Model file for the job. Use its own axes, mm. Give positions to 0.01 mm unless a question says otherwise; leave off trailing zeros. Loops run counter-clockwise (first coordinate to the right, second up) from the corner with the lowest first, then second, coordinate; pieces in that order, holes last. Notation, with made-up numbers: (4.5, 9) - (29.5, 9) arc R23 ccw to (29.5, 19) - close; hole circle Ø1 at (-0.5, -12.5). An arc over 180 degrees is marked (long way). Use a Markdown table: item, result.
from build123d import *

# Parameters (mm, degrees)
SKETCH_1_W      = 6
SKETCH_1_H      = 6
EXTRUDE_1_DEPTH = 20
HOLE_WIZARD_1_D = 2.5
HOLE_WIZARD_2_D = 2.5
CHAMFER_1_SIZE  = 0.3


with BuildPart() as part:
    # 草图1 → 凸台-拉伸1 (new, symmetric)
    with BuildSketch(Plane.XY):
        Rectangle(SKETCH_1_W, SKETCH_1_H)
    extrude(amount=EXTRUDE_1_DEPTH, both=True)

    # Hole Wizard 1 (through all)
    with Locations(Plane.ZY.offset(3)):
        with Locations((-15, 0), (5, 0)):
            Hole(HOLE_WIZARD_1_D / 2)

    # Hole Wizard 2 (through all)
    with Locations(Plane(origin=(0, 3, 0), x_dir=(1, 0, 0), z_dir=(0, 1, 0))):
        with Locations((0, 5), (0, -15)):
            Hole(HOLE_WIZARD_2_D / 2)

    # 倒角1
    chamfer_1_edges = [part.edges().sort_by_distance(p)[0] for p in [
        (-3, 0, 20),
        (0, -3, 20),
        (3, 0, 20),
        (0, -3, -20),
        (-3, 0, -20),
        (0, 3, -20),
        (3, 0, -20),
        (3, -3, 0),
        (-3, -3, 0),
        (-3, 3, 0),
        (3, 3, 0),
        (0, 3, 20),
    ]]
    chamfer(chamfer_1_edges, length=CHAMFER_1_SIZE)


solid = part.part
(1) Pin check, flat tip, straight feed: P1, Ø1, axis at y = 0, z = 5.5, coming from the +X side. Stop position of the tip, or through.
Computed:
| item | result |
|---|---|
| P1 | through |
(2) Drill centre lines: probe 1 along Z at (x, y) = (0, 1.85); probe 2 along X at (y, z) = (0.25, -5); probe 3 along Z at (x, y) = (1.5, 1). Where is each one in solid material? Low to high. Write a range as [from, to].
Computed:
| item | result |
|---|---|
| probe 1 | [-20, -6.25], [-3.75, 13.75], [16.25, 20] |
| probe 2 | [-3, -1.25], [1.25, 3] |
| probe 3 | [-20, -15.75], [-14.25, 4.25], [5.75, 20] |
(3) Slice it at B-B, the plane y = 0. Write the cut outline in (x, z).
Computed:
| item | result |
|---|---|
| outline | (-3, -19.7) - (-2.7, -20) - (2.7, -20) - (3, -19.7) - (3, -16.25) - (-3, -16.25) - close; (-3, -13.75) - (3, -13.75) - (3, 3.75) - (-3, 3.75) - close; (-3, 6.25) - (3, 6.25) - (3, 19.7) - (2.7, 20) - (-2.7, 20) - (-3, 19.7) - close; hole circle Ø2.5 at (0, -5); hole circle Ø2.5 at (0, 15) |
(4) Slice it at D-D, the plane y = -2. Write the cut outline in (x, z), plus the area to 3 significant figures.
Computed:
| item | result |
|---|---|
| outline | (-3, -19.7) - (-2.7, -20) - (2.7, -20) - (3, -19.7) - (3, 19.7) - (2.7, 20) - (-2.7, 20) - (-3, 19.7) - close; hole circle Ø2.5 at (0, -5); hole circle Ø2.5 at (0, 15) |
| area | 230 mm² |
(5) Mould opens along Z. For faces 1 (the cylindrical face through (0.16, -0.04, 13.76)), 2 (the cylindrical face through (0.04, 0.05, 6.25)), 3 (the flat face through (0, 3, 0)), 4 (the flat face through (0, 0, 20)) say: pulls with the +Z half, pulls with the -Z half, needs draft (parallel to the pull), parting line crosses it, or undercut.
Computed:
| item | result |
|---|---|
| face 1 | undercut |
| face 2 | undercut |
| face 3 | needs draft |
| face 4 | pulls with the +Z half |
(6) Slice it at A-A, the plane x = -0.75. Write the cut outline in (y, z).
Computed:
| item | result |
|---|---|
| outline | (-3, -19.7) - (-2.7, -20) - (2.7, -20) - (3, -19.7) - (3, -6) - (-3, -6) - close; (-3, -4) - (3, -4) - (3, 14) - (-3, 14) - close; (-3, 16) - (3, 16) - (3, 19.7) - (2.7, 20) - (-2.7, 20) - (-3, 19.7) - close; hole circle Ø2.5 at (0, -15); hole circle Ø2.5 at (0, 5) |
(7) Slice it at C-C, the plane z = 15. Write the cut outline in (x, y).
Computed:
| item | result |
|---|---|
| outline | (-3, -2.7) - (-2.7, -3) - (-1.25, -3) - (-1.25, 3) - (-2.7, 3) - (-3, 2.7) - close; (1.25, -3) - (2.7, -3) - (3, -2.7) - (3, 2.7) - (2.7, 3) - (1.25, 3) - close |
